Could you check a few things on this model? Use its own coordinates, in mm. A direction names the side the tool comes from. Coordinates: 2 decimals unless noted, no trailing zeros. Loops run counter-clockwise (first coordinate to the right, second up) from the corner with the lowest first, then second, coordinate; pieces in that order, holes last.
from build123d import *

# Parameters (mm, degrees)
ESQUISSE1_W        = 150
ESQUISSE1_H        = 64
BOSS_EXTRU_1_DEPTH = 93
ESQUISSE2_W        = 30
ESQUISSE2_H        = 10
BOSS_EXTRU_2_DEPTH = 10


with BuildPart() as part:
    # Esquisse1 → Boss.-Extru.1 (new body)
    with BuildSketch(Plane(origin=(0, 0, 0), x_dir=(1, 0, 0), z_dir=(0, 1, 0))):
        with Locations((40.269148016, 0)):
            Rectangle(ESQUISSE1_W, ESQUISSE1_H)
    extrude(amount=BOSS_EXTRU_1_DEPTH)

    # Esquisse2 → Boss.-Extru.2 (add)
    with BuildSketch(Plane(origin=(0, 93, 0), x_dir=(1, 0, 0), z_dir=(0, 1, 0))):
        with Locations((90.269148016, -22)):
            Rectangle(ESQUISSE2_W, ESQUISSE2_H)
    boss_extru_2 = extrude(amount=BOSS_EXTRU_2_DEPTH)

    # Symétrie1: Boss.-Extru.2 across plane
    add(boss_extru_2.mirror(Plane.XY))


solid = part.part
(1) Imagine slicing it at B-B, the plane x = 98. Write out the boundary of the cut face in (y, z), and give its area (3 significant figures).
Answers:
outline: (0, -32) - (93, -32) - (93, -27) - (103, -27) - (103, -17) - (93, -17) - (93, 17) - (103, 17) - (103, 27) - (93, 27) - (93, 32) - (0, 32) - close
area: 6,150 mm2
(2) Imagine slicing it at A-A, the plane z = -24. Write out the boundary of the cut face in (x, y), and give its area (4 significant figures).
Answers:
outline: (-34.73, 0) - (115.27, 0) - (115.27, 93) - (105.27, 93) - (105.27, 103) - (75.27, 103) - (75.27, 93) - (-34.73, 93) - close
area: 14,250 mm2
(3) Imagine slicing it at D-D, the plane z = -1. Write out the boundary of the cut face in (x, y), and give its area (4 significant figures).
Answers:
outline: (-34.73, 0) - (115.27, 0) - (115.27, 93) - (-34.73, 93) - close
area: 13,950 mm2
(4) We'd pull the mould along Z, two halves only. Please class faces 1 (the face through (115.269, 46, 0)), 2 (the face through (90, 98, 27)), 3 (the face through (90, 98, -17)): +Z half, -Z half, draft (parallel to the pull), parting line (faces both ways), or undercut.
Answers:
face 1: draft
face 2: +Z half
face 3: undercut
(5) Which directions (+Z, -Z, +X, -X, +Y, -Y) give clear straight access to the entire face, cutting with the end or side of a thin tool? Please do faces 4 (the face through (105.269, 98, -22)), 5 (the face through (90, 98, -27)), 6 (the face through (90, 98, 17)).
Answers:
face 4: +Z, -Z, +X, +Y
face 5: -Z, +X, -X, +Y
face 6: +X, -X, +Y
(6) I need wall thicknesses on probe 1 along Z at (x, y) = (76.5, 94); probe 2 along Y at (x, z) = (27.5, -14). Which ranges of each line are inside material? Lowest first, please.
Answers:
probe 1: z = -27 to -17, 17 to 27
probe 2: y = 0 to 93
(7) For pin 1 (19 mm diameter, centred on x = 41, z = -1.5, fed in from +Y); pin 2 (5 mm diameter, centred on x = 84, y = 96.5, fed in from -Z); pin 3 (3 mm diameter, centred on y = 96.5, z = 21, fed in from -X), each with a flat end and sliding along its axis, tell me the tip position at first contact or that it passes through.
Answers:
pin 1: stops at y = 93
pin 2: stops at z = -27
pin 3: stops at x = 75.27
(8) Imagine slicing it at C-C, the plane x = 22.5. Write out the boundary of the cut face in (y, z).
Answers:
outline: (0, -32) - (93, -32) - (93, 32) - (0, 32) - close
